```python
from build123d import *

# Parameters (mm, degrees)
F0_W           = 20
F0_H           = 12
F0_W_2         = 1
F0_H_2         = 0.6
F1_DEPTH       = 4
F2_D           = 4.5
F2_CBORE_D     = 8.25
F2_CBORE_DEPTH = 3
F3_R           = 1
F4_DEPTH       = 3.8


with BuildPart() as f1:
    # F0 (on Top) → F1 (new body)
    with BuildSketch(Plane.XY):
        Rectangle(F0_W, F0_H)
        with Locations((5, -2.5)):
            Rectangle(F0_W_2, F0_H_2, mode=Mode.SUBTRACT)
        with Locations((5, 2.5)):
            Rectangle(F0_W_2, F0_H_2, mode=Mode.SUBTRACT)
        with Locations((5, -2.5)):
            Rectangle(F0_W_2, F0_H_2)
        with Locations((5, 2.5)):
            Rectangle(F0_W_2, F0_H_2)
    extrude(amount=F1_DEPTH)

    # F2 (through all)
    with Locations(Plane(origin=(0, 0, 0), x_dir=(1, 0, 0), z_dir=(0, 0, -1))):
        with Locations((-5, 0)):
            CounterBoreHole(F2_D / 2, F2_CBORE_D / 2, F2_CBORE_DEPTH)

    # F3
    f3_edges = [f1.edges().sort_by_distance(p)[0] for p in [
        (-10, 6, 2),
        (10, 6, 2),
        (-10, -6, 2),
        (10, -6, 2),
    ]]
    fillet(f3_edges, radius=F3_R)

    # F0 (on Top) → F4 (cut)
    with BuildSketch(Plane.XY):
        with Locations((5, -2.5)):
            Rectangle(F0_W_2, F0_H_2)
        with Locations((5, 2.5)):
            Rectangle(F0_W_2, F0_H_2)
    extrude(amount=F4_DEPTH, mode=Mode.SUBTRACT)


solid = f1.part
```
For this review, take the finished solid that the model builds, in its own axes (mm). A direction names the side the tool comes from. Coordinates: 2 decimals unless noted, no trailing zeros. Write each loop counter-clockwise with the first axis right and the second up, starting at its lowest first coordinate (ties: lowest second). Pieces come first, ordered by that corner, then holes. Notation, with made-up numbers: (80, -33) - (92, -33) arc R8 cw to (92, -21) - close; hole circle Ø1 at (-33, -9.75). An arc over 180 degrees is marked (long way). Put each result on its own line as item: value.
1. Add section A-A, the plane z = 2.55. Give the boundary of the cut face in (x, y) (3 decimals), then the cut area to 3 significant figures.
Values found:
outline: (-10, -5) arc R1 ccw to (-9, -6) - (9, -6) arc R1 ccw to (10, -5) - (10, 5) arc R1 ccw to (9, 6) - (-9, 6) arc R1 ccw to (-10, 5) - close; hole circle Ø8.25 at (-5, 0); hole (4.5, -2.8) - (5.5, -2.8) - (5.5, -2.2) - (4.5, -2.2) - close; hole (4.5, 2.2) - (5.5, 2.2) - (5.5, 2.8) - (4.5, 2.8) - close
area: 184 mm²
2. Wall thickness on probe 1 along Y at (x, z) = (-5, 3.3); probe 2 along X at (y, z) = (2.5, 0.35); probe 3 along Y at (x, z) = (-5, 1.15) (3 decimals): over which ranges is each line inside the solid? List them lowest first.
Values found:
probe 1: -6 to -2.25, 2.25 to 6
probe 2: -10 to -8.28, -1.72 to 4.5, 5.5 to 10
probe 3: -6 to -4.125, 4.125 to 6
3. Machinability: for faces 1 (the flat face through (5, 2.2, 2)), 2 (the cylindrical face through (9.699, 5.715, 2.028)), which of the approach directions +Z, -Z, +X, -X, +Y, -Y give a long, thin tool a straight path to every point of the face, cutting with its end or side? Answer none if there is none.
Values found:
face 1: -Z
face 2: +Z, -Z, +X, +Y
4. Mouldability with a two-part tool opening along Y and no side actions: class faces 3 (the flat face through (0, 6, 2)), 4 (the flat face through (-10, 0, 2)), 5 (the cylindrical face through (9.699, -5.715, 2.028)), 6 (the flat face through (5, -2.8, 2)) as released by +Y, released by -Y, zero draft, split by the parting line, or undercut.
Values found:
face 3: released by +Y
face 4: zero draft
face 5: released by -Y
face 6: undercut
5. For pin 1 (0.5 mm diameter, centred on x = 5, y = -2.5, fed in from -Z), flat-tipped, find the tip position at first contact; note if it passes through.
Values found:
pin 1: z = 3.8
6. Add section B-B, the plane y = 0. Give the boundary of the cut face in (x, z) (3 decimals), then the cut area to 4 significant figures.
Values found:
outline: (-10, 0) - (-9.125, 0) - (-9.125, 3) - (-7.25, 3) - (-7.25, 4) - (-10, 4) - close; (-2.75, 3) - (-0.875, 3) - (-0.875, 0) - (10, 0) - (10, 4) - (-2.75, 4) - close
area: 50.75 mm²
7. Add section C-C, the plane x = -5. Give the boundary of the cut face in (y, z) (3 decimals), then the cut area to 4 significant figures.
Values found:
outline: (-6, 0) - (-4.125, 0) - (-4.125, 3) - (-2.25, 3) - (-2.25, 4) - (-6, 4) - close; (2.25, 3) - (4.125, 3) - (4.125, 0) - (6, 0) - (6, 4) - (2.25, 4) - close
area: 18.75 mm²
